Part model, mm, in its own coordinate system. Round coordinates to 2 decimals unless told otherwise and drop trailing zeros. Loops run counter-clockwise (first coordinate to the right, second up) from the corner with the lowest first, then second, coordinate; pieces in that order, holes last.
Solid Edge part; units mm, degrees
sketch "Sketch1" plane through (0, 0, 0) normal (0, -1, 0) x (1, 0, 0)
  line L0 (75, 12.5) -> (-75, 12.5)
  line L1 (-75, -12.5) -> (75, -12.5)
  arc A0 (-75, -12.5) -> (-75, 12.5) centre (-75, 0) cw
  arc A1 (75, 12.5) -> (75, -12.5) centre (75, 0) cw
  circle A2 centre (-75, 0) radius 4
  circle A3 centre (75, 0) radius 4
  circle A4 centre (0, 0) radius 3
extrude "ExtrudedProtrusion_2" add sketch "Sketch1" against normal blind 5
properties material "Polycarbonate( 20-40% Glass Fiber)"
1) Slice it at B-B, the plane x = 0. Give the cut face in (y, z), then the cut area to 3 significant figures.
Values:
outline: (0, -12.5) - (5, -12.5) - (5, -3) - (0, -3) - close; (0, 3) - (5, 3) - (5, 12.5) - (0, 12.5) - close
area: 95.0 mm2
2) Slice it at D-D, the plane z = 6.25. Give the cut face in (x, y), then the cut area to 3 significant figures.
Values:
outline: (-85.83, 0) - (85.83, 0) - (85.83, 5) - (-85.83, 5) - close
area: 858 mm2
3) Wall check: line 1 along X through (y, z) = (3.55, -1.5); line 2 along Z through (x, y) = (-75, 1.75); line 3 along Z through (x, y) = (0, 3.55). Give the ranges that are in metal, low to high.
Values:
line 1: x = -87.41 to -78.71, -71.29 to -2.6, 2.6 to 71.29, 78.71 to 87.41
line 2: z = -12.5 to -4, 4 to 12.5
line 3: z = -12.5 to -3, 3 to 12.5
4) Slice it at A-A, the plane z = 0. Give the cut face in (x, y), then the cut area to 3 significant figures.
Values:
outline: (-87.5, 0) - (-79, 0) - (-79, 5) - (-87.5, 5) - close; (-71, 0) - (-3, 0) - (-3, 5) - (-71, 5) - close; (3, 0) - (71, 0) - (71, 5) - (3, 5) - close; (79, 0) - (87.5, 0) - (87.5, 5) - (79, 5) - close
area: 765 mm2
5) Mould opens along X. For faces 1 (the face through (1, 2, 12.5)), 2 (the face through (-79, 2, 0)), 3 (the face through (-87.497, 2.465, 0.275)) say: released by +X, released by -X, zero draft, split by the parting line, or undercut.
Values:
face 1: zero draft
face 2: undercut
face 3: released by -X
6) Slice it at C-C, the plane y = 3.2. Give the cut face in (x, z).
Values:
outline: (-75, -12.5) - (75, -12.5) arc R12.5 ccw to (75, 12.5) - (-75, 12.5) arc R12.5 ccw to start; hole circle Ø8 at (-75, 0); hole circle Ø6 at (0, 0); hole circle Ø8 at (75, 0)
7) Drop flat-ended pins along their axis: pin 1 Ø7 at (x, z) = (-75, 0) entering from +Y; pin 2 Ø1 at (y, z) = (1.5, 1) entering from -X. Give the stop position or say it passes through.
Values:
pin 1: passes through
pin 2: stops at x = -87.49
